The figure shows three views and two pictorial views of one solid part (mm, origin at its lowest corner). Answer the questions. A direction names the side the tool comes from. Round coordinates to 2 decimals unless told otherwise and drop trailing zeros. Order: outer loops, then holes, each group sorted by start corner. A loop starts at its lowest first (then second) coordinate and runs counter-clockwise, first axis right, second up. Notation, with made-up numbers: (48, -38) - (105, -38) arc R32 ccw to (105, -10) - close; hole circle Ø6 at (20.25, -32). An arc over 180 degrees is marked (long way). Answer as a JSON object with one key per item and string values. Group by question number.
Q1. A cutting plane is placed at C-C on x = 22. Determine the outline of the cut face in (y, z).
Q2. A cutting plane is placed at D-D on y = 9. Determine the outline of the cut face in (x, z).
Q3. A cutting plane is placed at A-A on y = 6.5. Determine the outline of the cut face in (x, z).
Q4. Consider line 1 (Z direction, x = 10, y = 6.25) (1 decimal); line 2 (X direction, y = 8.5, z = 2); line 3 (Y direction, x = 1.5, z = 5.5). Determine where each line is inside the solid, lowest interval first.
Q5. The mould has two halves that part along Y. Classify the marked faces 3, 4 and 5: pulls with the +Y half, pulls with the -Y half, needs draft (parallel to the pull), parting line crosses it, or undercut.
Q6. A tool of negligible diameter and unlimited length cuts with its end or side. For the marked faces 1 and 2, from which of +Z, -Z, +X, -X, +Y, -Y can it reach the whole face along a straight path? Write none if from no direction.
Q7. Given pin 1 Ø2.5 at (y, z) = (5.99, 3.73) entering from +X; pin 2 Ø1.6 at (y, z) = (5.99, 14.86) entering from -X; pin 3 Ø3 at (y, z) = (5.99, 7.44) entering from -X; pin 4 Ø1 at (y, z) = (8.5, 12) entering from +X, each flat-ended and moving along its own axis, determine where each tip first touches the part or whether it passes through.
Q8. A cutting plane is placed at B-B on z = 14.5. Determine the outline of the cut face in (x, y) (1 decimal), and give its area (3 significant figures).
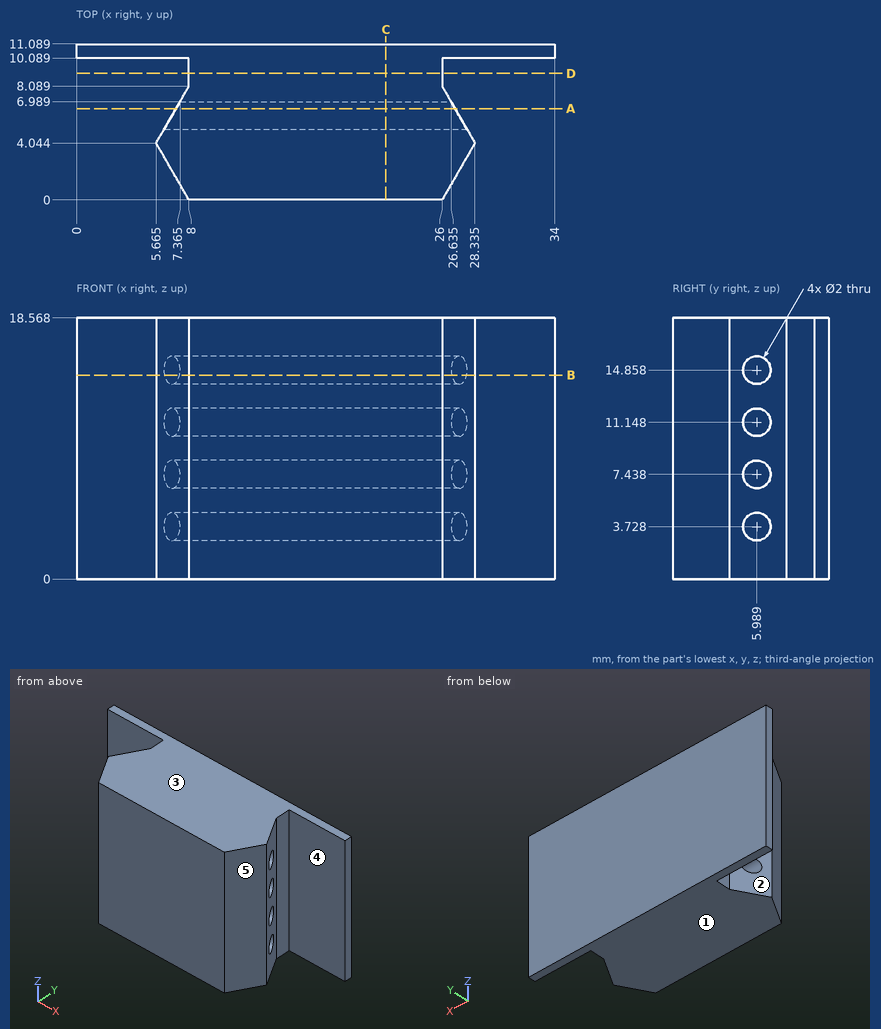
Result set:
{
 "1": {"outline": "(0, 0) - (11.09, 0) - (11.09, 18.57) - (0, 18.57) - close; hole circle Ø2 at (5.99, 3.73); hole circle Ø2 at (5.99, 7.44); hole circle Ø2 at (5.99, 11.15); hole circle Ø2 at (5.99, 14.86)"},
 "2": {"outline": "(8, 0) - (26, 0) - (26, 18.57) - (8, 18.57) - close"},
 "3": {"outline": "(7.08, 0) - (26.92, 0) - (26.92, 2.87) - (7.08, 2.87) - close; (7.08, 4.59) - (26.92, 4.59) - (26.92, 6.58) - (7.08, 6.58) - close; (7.08, 8.3) - (26.92, 8.3) - (26.92, 10.29) - (7.08, 10.29) - close; (7.08, 12.01) - (26.92, 12.01) - (26.92, 14) - (7.08, 14) - close; (7.08, 15.72) - (26.92, 15.72) - (26.92, 18.57) - (7.08, 18.57) - close"},
 "4": {"line 1": "z = 0 to 2.8, 4.7 to 6.5, 8.4 to 10.2, 12.1 to 13.9, 15.8 to 18.6", "line 2": "x = 8 to 26", "line 3": "y = 10.09 to 11.09"},
 "5": {"face 3": "needs draft", "face 4": "undercut", "face 5": "pulls with the -Y half"},
 "6": {"face 1": "-Z, +X, -X, +Y, -Y", "face 2": "+Z, -Z, -X"},
 "7": {"pin 1": "stops at x = 27.93", "pin 2": "passes through", "pin 3": "stops at x = 5.92", "pin 4": "stops at x = 26.05"},
 "8": {"outline": "(0, 10.1) - (8, 10.1) - (8, 8.1) - (7.3, 6.9) - (26.7, 6.9) - (26, 8.1) - (26, 10.1) - (34, 10.1) - (34, 11.1) - (0, 11.1) - close; (5.7, 4) - (8, 0) - (26, 0) - (28.3, 4) - (27.8, 5.1) - (6.2, 5.1) - close", "area": "196 mm²"}
}
